Part model, mm, in its own coordinate system. A direction names the side the tool comes from. Give positions to 0.01 mm unless a question says otherwise; leave off trailing zeros. Order: outer loops, then holes, each group sorted by start corner. A loop starts at its lowest first (then second) coordinate and runs counter-clockwise, first axis right, second up. Notation, with made-up numbers: (-30.75, -39.75) -> (1.25, -39.75) arc R19 cw to (1.25, -12.75) -> close; hole circle Ø2 at (41, -18). An arc over 180 degrees is marked (long way). Write item = value, one per line. Start each with the question number.
(1) Which spindle directions (+Z, -Z, +X, -X, +Y, -Y) get a long thin tool onto all of the face, cutting with end or side? Do faces 1 (the flat face through (60.364, -6, 20)), 2 (the flat face through (29.642, -7, 20)), 3 (the flat face through (114.808, 10, 28)). Say none if no direction does.
(2) Saw through at B-B, the plane y = -16.5. List the corners of the cut face in (x, z), then the cut area to 3 significant figures.
(3) Two-plate mould, pull along Y, no slides. Class faces 4 (the flat face through (36, 1, 39.751)), 5 (the cylindrical face through (52.34, -16.25, 20.15)), 6 (the flat face through (57, 19.939, 22)), 7 (the flat face through (15, 0, 20)): pulls with the +Y half, pulls with the -Y half, needs draft (parallel to the pull), parting line crosses it, or undercut.
(4) Probe line 1 along Y through (x, z) = (64, 9.5); line 2 along Z through (x, y) = (25, 1); line 3 along X through (y, z) = (-4.5, 19). List the from-to ranges inside material, lowest first. Write a range as from..to.
(5) Flat gauge pins, fed straight in: pin 1 (14 mm diameter, centred on y = -9.5, z = 22.5, fed in from +X); pin 2 (12 mm diameter, centred on x = 99, z = 15, fed in from -Y); pin 3 (10 mm diameter, centred on x = 40, y = -21, fed in from +Z). Where does each tip first touch, or does it go through?
(6) Saw through at D-D, the plane x = 25. List the corners of the cut face in (y, z).
(7) Saw through at A-A, the plane z = 17.5. List the corners of the cut face in (x, y) (1 decimal).
(8) Saw through at C-C, the plane y = 10. List the corners of the cut face in (x, z).
from build123d import *

# Parameters (mm, degrees)
F1_DEPTH      = 56.4388
F2_W          = 64.008
F2_H          = 16.6878
F3_DEPTH      = 25.4
F3_DEPTH_BACK = 58.166
F4_R          = 12.7
F6_DEPTH      = 19.939
F7_R          = 7.9375
F8_DEPTH      = 39.751


with BuildPart() as f1:
    # F0 (on Top) → F1 (new body)
    with BuildSketch(Plane.XY):
        with BuildLine():
            Line((0, 19.939), (0, 0))
            Line((0, 0), (29.6418, 0))
            Line((29.6418, 0), (29.6418, -13.208))
            ThreePointArc((29.6418, -13.208), (45.3057061406, -28.5721314673), (60.36432694, -12.6142985648))
            Line((60.36432694, -12.6142985648), (60.36432694, 0))
            Line((60.36432694, 0), (114.808, 0))
            Line((114.808, 0), (114.808, 19.939))
            Line((114.808, 19.939), (0, 19.939))
        make_face()
    extrude(amount=F1_DEPTH)

    # F2 (on Front) → F3 (cut, two sides)
    with BuildSketch(Plane.XZ) as f3_sk:
        with Locations((32.004, 48.0949)):
            Rectangle(F2_W, F2_H)
    extrude(amount=-F3_DEPTH, mode=Mode.SUBTRACT)
    extrude(f3_sk.sketch, amount=F3_DEPTH_BACK, mode=Mode.SUBTRACT)

    # F4
    f4_edges = [f1.edges().sort_by_distance(p)[0] for p in [
        (114.808, 9.9695, 56.4388),
        (114.808, 9.9695, 0),
        (64.008, 9.9695, 56.4388),
        (0, 9.9695, 39.751),
        (0, 9.9695, 0),
    ]]
    fillet(f4_edges, radius=F4_R)

    # F5 (on Front) → F6 (join, through all)
    with BuildSketch(Plane.XZ):
        with BuildLine():
            Line((60.36432694, 39.751), (60.3758, 39.751))
            Line((60.3758, 39.751), (64.008, 39.751))
            Line((64.008, 39.751), (64.008, 43.7388))
            ThreePointArc((64.008, 43.7388), (64.2020932514, 45.9506536109), (64.7784403774, 48.0949))
            ThreePointArc((64.7784403774, 48.0949), (60.1278755342, 42.0439718459), (52.8488807547, 39.751))
            Line((52.8488807547, 39.751), (60.36432694, 39.751))
        make_face()
    extrude(amount=-F6_DEPTH)

    # F7 (on face) → F8 (cut, through all)
    with BuildSketch(Plane.XY.offset(39.751)):
        with Locations((45.0088, -13.208)):
            Circle(F7_R)
    extrude(amount=-F8_DEPTH, mode=Mode.SUBTRACT)


solid = f1.part
Results list:
q1.face_1 = +Z, -Z, +X, -Y
q1.face_2 = +Z, -Z, -X, -Y
q1.face_3 = +Z, -Z, +X, +Y, -Y
q2.outline = (30, 0) -> (37.79, 0) -> (37.79, 39.75) -> (30, 39.75) -> close; (52.23, 0) -> (60.02, 0) -> (60.02, 39.75) -> (52.23, 39.75) -> close
q2.area = 619 mm^2
q3.face_4 = needs draft
q3.face_5 = undercut
q3.face_6 = pulls with the +Y half
q3.face_7 = pulls with the -Y half
q4.line_1 = 0..19.94
q4.line_2 = 0..39.75
q4.line_3 = 29.64..60.36
q5.pin_1 = 60.38
q5.pin_2 = 0
q5.pin_3 = 39.75
q6.outline = (0, 0) -> (19.94, 0) -> (19.94, 39.75) -> (0, 39.75) -> close
q7.outline = (0, 0) -> (29.6, 0) -> (29.6, -13.2) arc R15.4 ccw (long way) to (60.4, -12.6) -> (60.4, 0) -> (114.8, 0) -> (114.8, 19.9) -> (0, 19.9) -> close; hole circle Ø15.9 at (45, -13.2)
q8.outline = (0, 12.7) arc R12.7 ccw to (12.7, 0) -> (102.11, 0) arc R12.7 ccw to (114.81, 12.7) -> (114.81, 43.74) arc R12.7 ccw to (102.11, 56.44) -> (76.71, 56.44) arc R12.7 ccw to (64.78, 48.09) arc R12.7 cw to (52.85, 39.75) -> (12.7, 39.75) arc R12.7 ccw to (0, 27.05) -> close
